Read the model definition and answer for the solid it produces. Units are mm, in the model's axes. Face numbers are marked on the shaded views. A direction names the side the tool comes from. Round coordinates to 2 decimals unless told otherwise and drop trailing zeros. Loops run counter-clockwise (first coordinate to the right, second up) from the corner with the lowest first, then second, coordinate; pieces in that order, holes last. Notation, with made-up numbers: (-14, 48) - (32, 48) arc R14 ccw to (32, 59) - close; hole circle Ø4 at (27.5, -17). An arc over 180 degrees is marked (long way). Use one line per item in the form item = value. Start each with the question number.
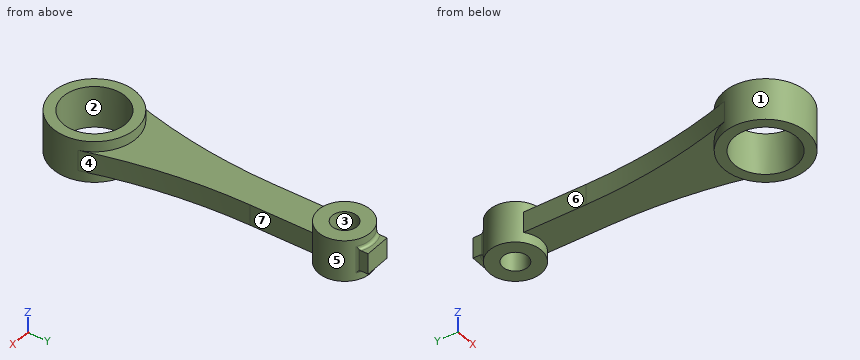
```python
from build123d import *

# Parameters (mm, degrees)
SKETCH3_R             = 20
SKETCH3_R_2           = 15
BOSS_EXTRUDE3_DEPTH   = 10
SKETCH3_R_3           = 12.5
SKETCH3_R_4           = 6
BOSS_EXTRUDE3_2_DEPTH = 10
BOSS_EXTRUDE4_DEPTH   = 5
BOSS_EXTRUDE5_DEPTH   = 5
FILLET1_R             = 1.5


with BuildPart() as part:
    # Sketch3 → Boss-Extrude3 (new body, symmetric)
    with BuildSketch(Plane.XY):
        Circle(SKETCH3_R)
        Circle(SKETCH3_R_2, mode=Mode.SUBTRACT)
    extrude(amount=BOSS_EXTRUDE3_DEPTH, both=True)



with BuildPart() as body_2:
    # Sketch3 → Boss-Extrude3 2 (new body, symmetric)
    with BuildSketch(Plane.XY):
        with Locations((0, 120)):
            Circle(SKETCH3_R_3)
        with Locations((0, 120)):
            Circle(SKETCH3_R_4, mode=Mode.SUBTRACT)
    extrude(amount=BOSS_EXTRUDE3_2_DEPTH, both=True)


with BuildPart() as part_1:
    add(part.part)

    add(body_2.part)  # Boss-Extrude4 merges body 2
    # Sketch4 → Boss-Extrude4 (add, symmetric)
    with BuildSketch(Plane.XY):
        with BuildLine():
            Line((8, 110.395313644), (8, 80.395313644))
            ThreePointArc((8, 80.395313644), (10.797388085, 42.704875811), (19.128250996, 5.840377886))
            ThreePointArc((19.128250996, 5.840377886), (0, 20), (-19.128250996, 5.840377886))
            ThreePointArc((-19.128250996, 5.840377886), (-10.797388085, 42.704875811), (-8, 80.395313644))
            Line((-8, 80.395313644), (-8, 110.395313644))
            ThreePointArc((-8, 110.395313644), (0, 107.5), (8, 110.395313644))
        make_face()
    extrude(amount=BOSS_EXTRUDE4_DEPTH, both=True)

    # Sketch5 → Boss-Extrude5 (add, symmetric)
    with BuildSketch(Plane.XY):
        with BuildLine():
            Line((-6.25, 135.825317547), (-6.25, 130.825317547))
            ThreePointArc((-6.25, 130.825317547), (0, 132.5), (6.25, 130.825317547))
            Line((6.25, 130.825317547), (6.25, 135.825317547))
            Line((6.25, 135.825317547), (-6.25, 135.825317547))
        make_face()
    extrude(amount=BOSS_EXTRUDE5_DEPTH, both=True)

    # Fillet1
    fillet1_edges = [part_1.edges().sort_by_distance(p)[0] for p in [
        (0, 132.5, -5),
        (-6.25, 130.825317547, 0),
        (6.25, 130.825317547, 0),
        (0, 132.5, 5),
    ]]
    fillet(fillet1_edges, radius=FILLET1_R)


solid = part_1.part
```
1) A cutting plane is placed at D-D on z = 2.25. Write down the section's boundary in (x, y), plus the area to 3 significant figures.
2) Flat-ended cylindrical pins translate along their axes: pin 1 (3.5 mm diameter, centred on x = 1.5, y = 134.5, fed in from -Z); pin 2 (6 mm diameter, centred on x = 4.5, z = -2.5, fed in from -Y); pin 3 (4.5 mm diameter, centred on y = 134.5, z = 0, fed in from -X); pin 4 (2.5 mm diameter, centred on x = 0.5, y = 133.5, fed in from +Z). Find the tip coordinate at first contact, or state that the pin passes through.
3) A cutting plane is placed at B-B on z = 8. Write down the section's boundary in (x, y), plus the area to 3 significant figures.
4) For the marked faces 5, 6 and 7, determine the directions among +Z, -Z, +X, -X, +Y, -Y from which every point of the face is accessible in a straight line to the end or side of a thin tool.
5) A cutting plane is placed at C-C on x = 0. Write down the section's boundary in (y, z), plus the area to 3 significant figures.
6) Determine the mould class of the marked faces 1, 2, 3 and 4 for opening direction X: +X half, -X half, draft (parallel to the pull), parting line (faces both ways), or undercut.
7) Straight lines are drawn through the part: line 1 (Y direction, x = 0, z = 3.5); line 2 (Y direction, x = -5, z = -0.5); line 3 (Z direction, x = 7.5, y = 26). For each, find the intervals that lie inside material, in ascending order. Write a range as from..to.
8) A cutting plane is placed at A-A on y = 0. Write down the section's boundary in (x, z), plus the area to 3 significant figures.
Checks:
q1.outline = (-19.13, 5.84) arc R20 ccw (long way) to (19.13, 5.84) arc R255.31 cw to (8, 80.4) - (8, 110.4) arc R12.5 ccw to (6.92, 130.41) arc R1.5 cw to (6.25, 131.66) - (6.25, 135.83) - (-6.25, 135.83) - (-6.25, 131.66) arc R1.5 cw to (-6.92, 130.41) arc R12.5 ccw to (-8, 110.4) - (-8, 80.4) arc R255.31 cw to start; hole circle Ø30 at (0, 0); hole circle Ø12 at (0, 120)
q1.area = 2,770 mm²
q2.pin_1 = -5.56
q2.pin_2 = -19.94
q2.pin_3 = -6.25
q2.pin_4 = 10
q3.outline = circle Ø40 at (0, 0); circle Ø25 at (0, 120); hole circle Ø30 at (0, 0); hole circle Ø12 at (0, 120)
q3.area = 928 mm²
q4.face_5 = none
q4.face_6 = +Z, -Z, -X
q4.face_7 = +Z, -Z, +X
q5.outline = (-20, -10) - (-15, -10) - (-15, 10) - (-20, 10) - close; (15, -10) - (20, -10) - (20, -5) - (107.5, -5) - (107.5, -10) - (114, -10) - (114, 10) - (107.5, 10) - (107.5, 5) - (20, 5) - (20, 10) - (15, 10) - close; (126, -10) - (132.5, -10) - (132.5, -6.5) arc R1.5 cw to (134, -5) - (135.83, -5) - (135.83, 5) - (134, 5) arc R1.5 cw to (132.5, 6.5) - (132.5, 10) - (126, 10) - close
q5.area = 1,370 mm²
q6.face_1 = parting line
q6.face_2 = undercut
q6.face_3 = undercut
q6.face_4 = +X half
q7.line_1 = -20..-15, 15..114, 126..135.83
q7.line_2 = -19.36..-14.14, 14.14..116.68, 123.32..135.83
q7.line_3 = -5..5
q8.outline = (-20, -10) - (-15, -10) - (-15, 10) - (-20, 10) - close; (15, -10) - (20, -10) - (20, 10) - (15, 10) - close
q8.area = 200 mm²
